Geometry: final body of the model. Coordinates: model frame, mm. A direction names the side the tool comes from. Coordinates: 2 decimals unless noted, no trailing zeros. Order: outer loops, then holes, each group sorted by start corner. A loop starts at its lowest first (then second) coordinate and runs counter-clockwise, first axis right, second up. Notation, with made-up numbers: M 42.5,83.5 L 64.5,83.5 A27 cw 64.5,121.5 Z; hole C 42.25,62 d7. An arc over 180 degrees is marked long. Use CSV: the item, a comma, the result in double quotes. Start each with the question number.
1. Section query B-B on x = 280.5. Return the cut outline in (y, z).
2. Section query A-A on y = 260. Return the cut outline in (x, z).
3. Material intervals for line 1 (Y direction, x = 289.5, z = 339.25); line 2 (Y direction, x = 287, z = 338.25); line 3 (X direction, y = 308.25, z = 338.5), sorted ascending.
4. Pull-direction query (X, two-part tool) for faces 1 (the flat face through (300, 200, 340.2)), 2 (the flat face through (279, 234, 333.5)); classes: pulls with the +X half, pulls with the -X half, needs draft (parallel to the pull), parting line crosses it, or undercut.
5. First-contact query: P1, Ø5, axis at y = 175, z = 340.5, coming from the +X side; P2, Ø3, axis at x = 305, y = 300, coming from the -Z side; P3, Ø1, axis at x = 313, y = 223, coming from the -Z side; P4, Ø2.5, axis at x = 309.5, z = 346.5, coming from the +Y side. Flat tips, straight axial feed; report the tip coordinate or a pass-through.
6. Section query D-D on y = 200. Return the cut outline in (x, z).
7. Section query C-C on y = 240. Return the cut outline in (x, z).
8. Set-up query: faces 3 (the flat face through (302.2, 200.1, 333.5)), 4 (the cylindrical face through (303.3, 260, 346)), 5 (the cylindrical face through (291.156, 178.11, 343.486)). Return all of +Z, -Z, +X, -X, +Y, -Y with unobstructed straight access to the full face (end or side cutting, diameter ignored); none if empty.
from build123d import *

# Parameters (mm, degrees)
SKETCH1_R           = 6
SKETCH1_R_2         = 1.45
BOSS_EXTRUDE1_DEPTH = 3
SKETCH2_R           = 20
SKETCH2_R_2         = 1.45
BOSS_EXTRUDE2_DEPTH = 2
SKETCH3_R           = 12
SKETCH3_R_2         = 6
BOSS_EXTRUDE3_DEPTH = 2
BOSS_EXTRUDE4_DEPTH = 11
SKETCH5_R           = 5.05
BOSS_EXTRUDE5_DEPTH = 11
SKETCH6_R           = 5.05
BOSS_EXTRUDE6_DEPTH = 11
SKETCH7_R           = 5.05
BOSS_EXTRUDE7_DEPTH = 11
SKETCH8_R           = 5.05
BOSS_EXTRUDE8_DEPTH = 11
SKETCH9_R           = 2.05
CUT_EXTRUDE1_DEPTH  = 6.7
SKETCH10_R          = 7.6
CUT_EXTRUDE2_DEPTH  = 5
SKETCH11_R          = 8.05
CUT_EXTRUDE3_DEPTH  = 4.5


with BuildPart() as part:
    # Sketch1 → Boss-Extrude1 (new body)
    with BuildSketch(Plane.XY.offset(344.5)):
        with BuildLine():
            Line((276.003127371, 300.387432585), (273.904807661, 170.421310226))
            ThreePointArc((273.904807661, 170.421310226), (300, 143.901406829), (326.095192339, 170.421310226))
            Line((326.095192339, 170.421310226), (323.996872629, 300.387432585))
            ThreePointArc((323.996872629, 300.387432585), (300, 324), (276.003127371, 300.387432585))
        make_face()
        with Locations((300, 170)):
            Circle(SKETCH1_R, mode=Mode.SUBTRACT)
        with Locations((300, 313.5)):
            Circle(SKETCH1_R_2, mode=Mode.SUBTRACT)
        with Locations((288.308657049, 293.25)):
            Circle(SKETCH1_R_2, mode=Mode.SUBTRACT)
        with Locations((311.691342951, 293.25)):
            Circle(SKETCH1_R_2, mode=Mode.SUBTRACT)
        with BuildLine():
            Line((305, 258.3), (314, 258.3))
            ThreePointArc((314, 258.3), (315.7, 260), (314, 261.7))
            Line((314, 261.7), (305, 261.7))
            ThreePointArc((305, 261.7), (303.3, 260), (305, 258.3))
        make_face(mode=Mode.SUBTRACT)
    extrude(amount=BOSS_EXTRUDE1_DEPTH)

    # Sketch2 → Boss-Extrude2 (add)
    with BuildSketch(Plane.XY.offset(342.5)):
        with Locations((300, 300)):
            Circle(SKETCH2_R)
        with Locations((300, 313.5)):
            Circle(SKETCH2_R_2, mode=Mode.SUBTRACT)
        with Locations((288.308657049, 293.25)):
            Circle(SKETCH2_R_2, mode=Mode.SUBTRACT)
        with Locations((311.691342951, 293.25)):
            Circle(SKETCH2_R_2, mode=Mode.SUBTRACT)
    extrude(amount=BOSS_EXTRUDE2_DEPTH)

    # Sketch3 → Boss-Extrude3 (add)
    with BuildSketch(Plane.XY.offset(342.5)):
        with Locations((300, 170)):
            Circle(SKETCH3_R)
        with Locations((300, 170)):
            Circle(SKETCH3_R_2, mode=Mode.SUBTRACT)
    extrude(amount=BOSS_EXTRUDE3_DEPTH)

    # Sketch4 → Boss-Extrude4 (add)
    with BuildSketch(Plane.XY.offset(333.5)):
        with BuildLine():
            Line((276.003127371, 300.387432585), (273.904807661, 170.421310226))
            ThreePointArc((273.904807661, 170.421310226), (300, 143.901406829), (326.095192339, 170.421310226))
            Line((326.095192339, 170.421310226), (323.996872629, 300.387432585))
            ThreePointArc((323.996872629, 300.387432585), (300, 324), (276.003127371, 300.387432585))
        make_face()
        with BuildLine():
            Line((282.510952348, 300.619041388), (277.9152372, 170.781711074))
            ThreePointArc((277.9152372, 170.781711074), (300, 147.901406829), (322.0847628, 170.781711074))
            Line((322.0847628, 170.781711074), (317.489047652, 300.619041388))
            ThreePointArc((317.489047652, 300.619041388), (300, 317.5), (282.510952348, 300.619041388))
        make_face(mode=Mode.SUBTRACT)
    extrude(amount=BOSS_EXTRUDE4_DEPTH)

    # Sketch5 → Boss-Extrude5 (add)
    with BuildSketch(Plane.XY.offset(333.5)):
        with Locations((314.289419162, 308.25)):
            Circle(SKETCH5_R)
    extrude(amount=BOSS_EXTRUDE5_DEPTH)

    # Sketch6 → Boss-Extrude6 (add)
    with BuildSketch(Plane.XY.offset(333.5)):
        with Locations((285.710580838, 308.25)):
            Circle(SKETCH6_R)
    extrude(amount=BOSS_EXTRUDE6_DEPTH)

    # Sketch7 → Boss-Extrude7 (add)
    with BuildSketch(Plane.XY.offset(333.5)):
        with Locations((300, 240)):
            Circle(SKETCH7_R)
    extrude(amount=BOSS_EXTRUDE7_DEPTH)

    # Sketch8 → Boss-Extrude8 (add)
    with BuildSketch(Plane.XY.offset(333.5)):
        with Locations((300, 200)):
            Circle(SKETCH8_R)
    extrude(amount=BOSS_EXTRUDE8_DEPTH)

    # Sketch9 → Cut-Extrude1 (cut)
    with BuildSketch(Plane.XY.offset(333.5)):
        with Locations(Location((314.289419162, 308.25, 0), (0, 0, 180))):
            Circle(SKETCH9_R)
        with Locations(Location((285.710580838, 308.25, 0), (0, 0, 180))):
            Circle(SKETCH9_R)
        with Locations(Location((300, 240, 0), (0, 0, 180))):
            Circle(SKETCH9_R)
        with Locations(Location((300, 200, 0), (0, 0, 180))):
            Circle(SKETCH9_R)
    extrude(amount=CUT_EXTRUDE1_DEPTH, mode=Mode.SUBTRACT)

    # Sketch10 → Cut-Extrude2 (cut)
    with BuildSketch(Plane.XY.offset(342.5)):
        with Locations((300, 300)):
            Circle(SKETCH10_R)
    extrude(amount=CUT_EXTRUDE2_DEPTH, mode=Mode.SUBTRACT)

    # Sketch11 → Cut-Extrude3 (cut)
    with BuildSketch(Plane.XY.offset(342.5)):
        with Locations((300, 170)):
            Circle(SKETCH11_R)
    extrude(amount=CUT_EXTRUDE3_DEPTH, mode=Mode.SUBTRACT)


solid = part.part
Results list:
1,outline,"M 152.65,333.5 L 159.6,333.5 L 159.6,344.5 L 243.81,344.5 L 243.81,333.5 L 313.99,333.5 L 313.99,347.5 L 152.65,347.5 Z"
2,outline,"M 275.35,333.5 L 281.07,333.5 L 281.07,344.5 L 303.3,344.5 L 303.3,347.5 L 275.35,347.5 Z; M 315.7,344.5 L 318.93,344.5 L 318.93,333.5 L 324.65,333.5 L 324.65,347.5 L 315.7,347.5 Z"
3,line 1,"y = 146.11 to 150.56, 304.91 to 311.59, 314 to 321.58"
3,line 2,"y = 147.37 to 152.13, 303.37 to 306.66, 309.84 to 320.17"
3,line 3,"x = 277.46 to 283.66, 287.76 to 290.76, 309.24 to 312.24, 316.34 to 322.54"
4,face 1,"undercut"
4,face 2,"needs draft"
5,P1,"stops at x = 326.06"
5,P2,"passes through"
5,P3,"stops at z = 344.5"
5,P4,"stops at y = 322.54"
6,outline,"M 274.38,333.5 L 278.95,333.5 L 278.95,344.5 L 294.95,344.5 L 294.95,333.5 L 297.95,333.5 L 297.95,340.2 L 302.05,340.2 L 302.05,333.5 L 305.05,333.5 L 305.05,344.5 L 321.05,344.5 L 321.05,333.5 L 325.62,333.5 L 325.62,347.5 L 274.38,347.5 Z"
7,outline,"M 275.03,333.5 L 280.37,333.5 L 280.37,344.5 L 294.95,344.5 L 294.95,333.5 L 297.95,333.5 L 297.95,340.2 L 302.05,340.2 L 302.05,333.5 L 305.05,333.5 L 305.05,344.5 L 319.63,344.5 L 319.63,333.5 L 324.97,333.5 L 324.97,347.5 L 275.03,347.5 Z"
8,face 3,"-Z, +X, -X, +Y, -Y"
8,face 4,"+Z, -Z"
8,face 5,"-Z"
